Verification items for the finished model (mm, model axes). A direction names the side the tool comes from. Coordinates: 2 decimals unless noted, no trailing zeros. Order: outer loops, then holes, each group sorted by start corner. A loop starts at its lowest first (then second) coordinate and runs counter-clockwise, first axis right, second up. Notation, with made-up numbers: M -38,-17.75 L 0,-17.75 A21 ccw 0,-5.75 Z; hole C -25,73 d9. An arc over 180 degrees is marked long. Write item = value, one per line.
Autodesk Fusion 360 part; units mm, degrees
sketch "スケッチ1" plane through (0, 0, 0) normal (0, 0, 1) x (1, 0, 0)
  line L0 (0, 0) -> (20, 0)
  line L1 (20, 0) -> (20, 20)
  line L2 (20, 20) -> (0, 20)
  line L3 (0, 20) -> (0, 0)
extrude "押し出し1" add sketch "スケッチ1" along normal blind 10.5
sketch "スケッチ2" plane through (0, 0, 10.5) normal (0, 0, 1) x (-1, 0, 0)
  line L0 (0, -20) -> (0, 0)
  line L1 (0, 0) -> (-20, 0)
  line L2 (-20, 0) -> (-20, -20)
  line L3 (-20, -20) -> (0, -20)
  line L4 (-7.5, -3) -> (-12.5, -3)
  line L5 (-12.5, -3) -> (-12.5, -6)
  line L6 (-12.5, -6) -> (-7.5, -6)
  line L7 (-7.5, -6) -> (-7.5, -3)
  line L8 (-6, -12.5) -> (-3, -12.5)
  line L9 (-3, -12.5) -> (-3, -7.5)
  line L10 (-3, -7.5) -> (-6, -7.5)
  line L11 (-6, -7.5) -> (-6, -12.5)
  dimension "d3" = 7.5
  dimension "d4" = 3
  dimension "d5" = 7.5
  dimension "d6" = 3
extrude "押し出し2" add sketch "スケッチ2" along normal blind 10.5 contours L4 L5 L6 L7 | L8 L9 L10 L11
sketch "スケッチ4" plane through (0, 0, 0) normal (0, 0, -1) x (1, 0, 0)
  line L0 (0, 0) -> (0, -20)
  line L1 (0, -20) -> (20, -20)
  line L2 (20, -20) -> (20, 0)
  line L3 (20, 0) -> (0, 0)
  line L4 (20, -20) -> (7, -20)
  line L5 (7, -20) -> (7, -8)
  line L6 (7, -8) -> (20, -8)
  line L7 (20, -8) -> (20, -20)
  dimension "d14" = 12
  dimension "d15" = 13
extrude "押し出し4" cut sketch "スケッチ4" against normal blind 18 contours L1 L2 L4 L5 L6 L7
fillet "フィレット1" radius 9 1 edges at (7, 8, 5.25)
extrude "押し出し5" add 1 faces at (11.1548, 2.7882, 0) along direction (0, 0, -1) blind 5
sketch "スケッチ3" plane through (20, 0, 0) normal (1, 0, 0) x (0, 1, 0)
  line L0 (8, 10.5) -> (0, 10.5)
  line L1 (0, 10.5) -> (0, -5)
  circle A0 centre (3, -2.5) radius 1.5
  line L2 (8, -5) -> (8, 10.5)
  line L3 (0, -5) -> (8, -5)
  dimension "d9" = 3
  dimension "d10" = 3
  dimension "d22" = 2.5
extrude "押し出し3" cut sketch "スケッチ3" against normal blind 22 contours A0
Item 1: Tool access check on faces 4 (the flat face through (7, 19, 3)), 5 (the flat face through (10, 3, 16)), 6 (the flat face through (10, 6, 16)). Record the directions out of +Z, -Z, +X, -X, +Y, -Y that give a thin tool (end or side, any length) a straight path to the whole face; none if there is none.
Report:
face_4 = +Z, -Z, +X, +Y
face_5 = +Z, +X, -X, -Y
face_6 = +Z, +X, -X, +Y
Item 2: Sectioned sample at B-B, the plane y = 5. Enter the section's corners in (x, z).
Report:
outline = M 0,-5 L 20,-5 L 20,10.5 L 12.5,10.5 L 12.5,21 L 7.5,21 L 7.5,10.5 L 0,10.5 Z
Item 3: Sectioned sample at A-A, the plane z = -2.5. Enter the section's corners in (x, y), then the cut area to 3 significant figures.
Report:
outline = M 0,0 L 20,0 L 20,1.5 L 0,1.5 Z; M 0,4.5 L 20,4.5 L 20,8 L 16,8 A9 cw 7,17 L 7,20 L 0,20 Z
area = 201 mm^2
Item 4: Scan lines: L1, parallel to Z at x = 15.75, y = 3; L2, parallel to Z at x = 9, y = 8.75; L3, parallel to Z at x = 14.5, y = 2. Record each from-to range of solid material in increasing order. Write a range as from..to.
Report:
L1 = -5..-4, -1..10.5
L2 = -5..10.5
L3 = -5..-3.62, -1.38..10.5
Item 5: Gauge pin test, flat ends, axial feed: pin 1 (5.5 mm diameter, centred on x = 10, z = 16, fed in from +Y); pin 2 (2.5 mm diameter, centred on x = 10.5, z = 15.5, fed in from -Y); pin 3 (4 mm diameter, centred on y = 9.5, z = 13.5, fed in from -X). Record the tip position at first contact, or that the pin passes through.
Report:
pin_1 = 6
pin_2 = 3
pin_3 = 3
Item 6: Sectioned sample at D-D, the plane x = 8.75. Enter the section's corners in (y, z).
Report:
outline = M 0,-5 L 11.67,-5 L 11.67,10.5 L 6,10.5 L 6,21 L 3,21 L 3,10.5 L 0,10.5 Z; hole C 3,-2.5 d3
Item 7: Release check for a two-part mould opening along Z. For faces 1 (the cylindrical face through (10.14, 3.806, -1.235)), 2 (the flat face through (6, 10, 16)), 3 (the flat face through (8, 8, -5)) record: pulls with the +Z half, pulls with the -Z half, needs draft (parallel to the pull), parting line crosses it, or undercut.
Report:
face_1 = undercut
face_2 = needs draft
face_3 = pulls with the -Z half
Item 8: Sectioned sample at C-C, the plane z = 8. Enter the section's corners in (x, y), then the cut area to 3 significant figures.
Report:
outline = M 0,0 L 20,0 L 20,8 L 16,8 A9 cw 7,17 L 7,20 L 0,20 Z
area = 261 mm^2
